Can you work these out from the drawing? Everything is in mm from the part's minimum corner. Coordinates: 2 decimals unless noted, no trailing zeros. Loops run counter-clockwise (first coordinate to the right, second up) from the corner with the lowest first, then second, coordinate; pieces in that order, holes last.
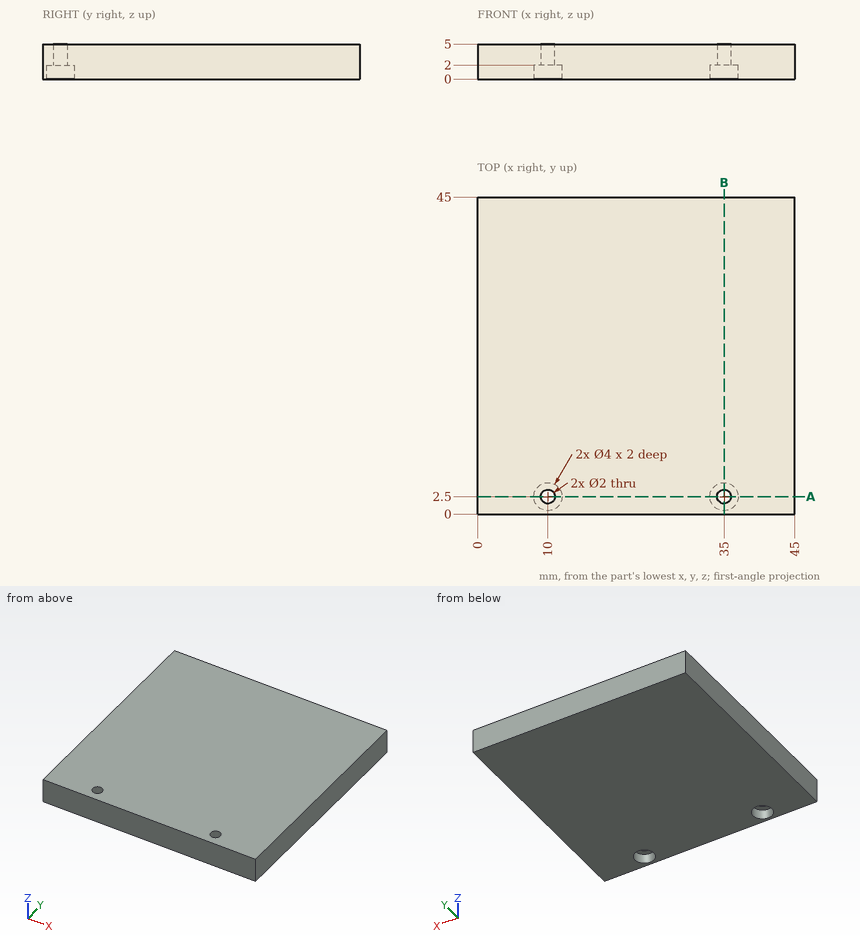
(1) For pin 1 (1.5 mm diameter, centred on x = 15, y = 31, fed in from -Z); pin 2 (2.5 mm diameter, centred on x = 10, y = 2.5, fed in from -Z), each with a flat end and sliding along its axis, tell me the tip position at first contact or that it passes through.
Answers:
pin 1: stops at z = 0
pin 2: stops at z = 2
(2) Imagine slicing it at A-A, the plane y = 2.5. Write out the boundary of the cut face in (x, z).
Answers:
outline: (0, 0) - (8, 0) - (8, 2) - (9, 2) - (9, 5) - (0, 5) - close; (11, 2) - (12, 2) - (12, 0) - (33, 0) - (33, 2) - (34, 2) - (34, 5) - (11, 5) - close; (36, 2) - (37, 2) - (37, 0) - (45, 0) - (45, 5) - (36, 5) - close
(3) Imagine slicing it at B-B, the plane x = 35. Write out the boundary of the cut face in (y, z).
Answers:
outline: (0, 0) - (0.5, 0) - (0.5, 2) - (1.5, 2) - (1.5, 5) - (0, 5) - close; (3.5, 2) - (4.5, 2) - (4.5, 0) - (45, 0) - (45, 5) - (3.5, 5) - close
(4) I need wall thicknesses on probe 1 along X at (y, z) = (2.5, 1.25); probe 2 along Y at (x, z) = (35, 3.85); probe 3 along Y at (x, z) = (10, 0.8). Which ranges of each line are inside material? Lowest first, please.
Answers:
probe 1: x = 0 to 8, 12 to 33, 37 to 45
probe 2: y = 0 to 1.5, 3.5 to 45
probe 3: y = 0 to 0.5, 4.5 to 45
